Could you check a few things on this model? Use its own coordinates, in mm. A direction names the side the tool comes from. Give positions to 0.01 mm unless a question says otherwise; leave off trailing zeros. Loops run counter-clockwise (first coordinate to the right, second up) from the corner with the lowest first, then second, coordinate; pieces in that order, holes last. Notation, with made-up numbers: M 32.25,4.5 L 71.25,4.5 A17 ccw 71.25,8.5 Z; hole C -18,-37.5 d10. An arc over 180 degrees is marked long. Return JSON: item names as keys, results as strings. Group by question number.
1. For pin 1 (3 mm diameter, centred on y = -4, z = -172.5, fed in from -X); pin 2 (1.5 mm diameter, centred on y = -48, z = 127.5, fed in from -X); pin 3 (3 mm diameter, centred on y = -63, z = -123.5, fed in from -X), each with a flat end and sliding along its axis, tell me the tip position at first contact or that it passes through.
2. If we section it at B-B (x = 0): Write out the boundary of the cut face in (y, z), plus the area to 3 significant figures.
3. If we section it at C-C (y = 20): Write out the boundary of the cut face in (x, z).
4. Please list where these lines run through material, in increasing order: line 1 (Z direction, x = 0, y = -71); line 2 (Z direction, x = 0, y = -83.25); line 3 (X direction, y = -71.5, z = -71).
5. If we section it at D-D (y = -77): Write out the boundary of the cut face in (x, z).
6. If we section it at A-A (z = 0): Write out the boundary of the cut face in (x, y).
7. If we mould it in two halves opening along X, with no side actions, what happens to faces 4 (the flat face through (-21, 63.5, 1)), 5 (the flat face through (93, 88.9, -45)), 6 (the cylindrical face through (-55.06, -0.71, -247.96))? For each: +X half, -X half, draft (parallel to the pull), parting line (faces both ways), or undercut.
8. For faces 1 (the flat face through (93, -88.9, -45)), 2 (the cylindrical face through (22.025, 76.378, -99.184)), 3 (the cylindrical face through (-22.025, -76.378, -99.184)), which set-ups out of +Z, -Z, +X, -X, +Y, -Y let a thin tool reach every point of the face, with its end or its side?
```python
from build123d import *

# Parameters (mm, degrees)
F0_R     = 254
F1_DEPTH = 88.9
F2_R     = 101.6
F3_DEPTH = 25.4
F4_R     = 101.6
F5_DEPTH = 25.4
F6_R     = 38.1
F7_R     = 12.7
F8_DEPTH = 177.8


with BuildPart() as f1:
    # F0 (on Front) → F1 (new body, symmetric)
    with BuildSketch(Plane.XZ):
        Circle(F0_R)
    extrude(amount=F1_DEPTH, both=True)

    # F2 (on face) → F3 (cut)
    with BuildSketch(Plane.XZ.offset(88.9)):
        Circle(F2_R)
    extrude(amount=-F3_DEPTH, mode=Mode.SUBTRACT)

    # F4 (on face) → F5 (cut)
    with BuildSketch(Plane(origin=(0, 88.9, 0), x_dir=(-1, 0, 0), z_dir=(0, 1, 0))):
        Circle(F4_R)
    extrude(amount=-F5_DEPTH, mode=Mode.SUBTRACT)

    # F6
    f6_edges = [f1.edges().sort_by_distance(p)[0] for p in [
        (-254, 88.9, 0),
        (-254, -88.9, 0),
    ]]
    fillet(f6_edges, radius=F6_R)

    # F7 (on face) → F8 (cut, symmetric)
    with BuildSketch(Plane(origin=(0, 63.5, 0), x_dir=(-1, 0, 0), z_dir=(0, 1, 0))):
        Circle(F7_R)
    extrude(amount=F8_DEPTH, both=True, mode=Mode.SUBTRACT)


solid = f1.part
```
Answer:
{
 "1": {"pin 1": "stops at x = -187.82", "pin 2": "stops at x = -220.11", "pin 3": "stops at x = -220.66"},
 "2": {"outline": "M -88.9,-215.9 A38.1 ccw -50.8,-254 L 50.8,-254 A38.1 ccw 88.9,-215.9 L 88.9,-101.6 L 63.5,-101.6 L 63.5,-12.7 L -63.5,-12.7 L -63.5,-101.6 L -88.9,-101.6 Z; M -88.9,101.6 L -63.5,101.6 L -63.5,12.7 L 63.5,12.7 L 63.5,101.6 L 88.9,101.6 L 88.9,215.9 A38.1 ccw 50.8,254 L -50.8,254 A38.1 ccw -88.9,215.9 Z", "area": "75,500 mm²"},
 "3": {"outline": "C 0,0 d508; hole C 0,0 d25.4"},
 "4": {"line 1": "z = -248.2 to -101.6, 101.6 to 248.2", "line 2": "z = -235.87 to -101.6, 101.6 to 235.87", "line 3": "x = -237.5 to -72.67, 72.67 to 237.5"},
 "5": {"outline": "C 0,0 d487.12; hole C 0,0 d203.2"},
 "6": {"outline": "M -254,-50.8 A38.1 ccw -215.9,-88.9 L -101.6,-88.9 L -101.6,-63.5 L -12.7,-63.5 L -12.7,63.5 L -101.6,63.5 L -101.6,88.9 L -215.9,88.9 A38.1 ccw -254,50.8 Z; M 12.7,-63.5 L 101.6,-63.5 L 101.6,-88.9 L 215.9,-88.9 A38.1 ccw 254,-50.8 L 254,50.8 A38.1 ccw 215.9,88.9 L 101.6,88.9 L 101.6,63.5 L 12.7,63.5 Z"},
 "7": {"face 4": "undercut", "face 5": "draft", "face 6": "parting line"},
 "8": {"face 1": "+Z, -Z, +X, -X, -Y", "face 2": "+Y", "face 3": "-Y"}
}
